Autodesk Fusion 360 part; units mm, degrees
sketch "Sketch1" plane through (0, 0, 0) normal (0, 0, 1) x (1, 0, 0)
  line L0 (0, 0) -> (49, 0)
  line L1 (49, 0) -> (49, 74)
  line L2 (49, 74) -> (0, 74)
  line L3 (0, 74) -> (0, 0)
extrude "Extrude1" add sketch "Sketch1" along normal blind 10
sketch "Sketch2" plane through (0, 0, 10) normal (0, 0, 1) x (-1, 0, 0)
  line L0 (0, -74) -> (0, 0)
  line L1 (0, 0) -> (-49, 0)
  line L2 (-49, 0) -> (-49, -74)
  line L3 (-49, -74) -> (0, -74)
  line L4 (-1.9, -72.1) -> (-47.1, -72.1)
  line L5 (-47.1, -72.1) -> (-47.1, -1.9)
  line L6 (-47.1, -1.9) -> (-1.9, -1.9)
  line L7 (-1.9, -1.9) -> (-1.9, -72.1)
extrude "Extrude2" cut sketch "Sketch2" against normal blind 9 contours L4 L5 L6 L7
sketch "Sketch3" plane through (0, 74, 0) normal (0, 1, 0) x (-1, 0, 0)
  line L0 (-49, 0) -> (0, 0)
  line L1 (0, 0) -> (0, 10)
  line L2 (0, 10) -> (-49, 10)
  line L3 (-49, 10) -> (-49, 0)
sketch "Sketch4" plane through (0, 74, 0) normal (0, 1, 0) x (-1, 0, 0)
  line L0 (-5, 5) -> (-19, 5)
  line L1 (-19, 5) -> (-19, 10)
  line L2 (-19, 10) -> (-5, 10)
  line L3 (-5, 10) -> (-5, 5)
extrude "Extrude3" cut sketch "Sketch4" against normal blind 6
sketch "Sketch5" plane through (0, 0, 0) normal (0, 1, 0) x (1, 0, 0)
sketch "Sketch6" plane through (0, 0, 0) normal (0, -1, 0) x (1, 0, 0)
  line L0 (0, 0) -> (49, 0)
  line L1 (49, 0) -> (49, 10)
  line L2 (49, 10) -> (0, 10)
  line L3 (0, 10) -> (0, 0)
  line L4 (6, 5) -> (19, 5)
  line L5 (19, 5) -> (19, 10)
  line L6 (19, 10) -> (6, 10)
  line L7 (6, 10) -> (6, 5)
extrude "Extrude4" cut sketch "Sketch6" against normal blind 6 contours L2 L4 L5 L6 L7
sketch "Sketch7" plane through (0, 0, 0) normal (-1, 0, 0) x (0, -1, 0)
  line L0 (-74, 0) -> (0, 0)
  line L1 (0, 0) -> (0, 10)
  line L2 (0, 10) -> (-74, 10)
  line L3 (-74, 10) -> (-74, 0)
  line L4 (-23, 11) -> (-47, 11)
  line L5 (-47, 11) -> (-47, 3)
  line L6 (-47, 3) -> (-23, 3)
  line L7 (-23, 3) -> (-23, 11)
extrude "Extrude5" cut sketch "Sketch7" against normal blind 3 contours L2 L5 L6 L7
sketch "Sketch8" plane through (0, 0, 1) normal (0, 0, 1) x (-1, 0, 0)
  line L0 (-1.9, -1.9) -> (-47.1, -1.9)
  line L1 (-47.1, -1.9) -> (-47.1, -72.1)
  line L2 (-47.1, -72.1) -> (-1.9, -72.1)
  line L3 (-1.9, -72.1) -> (-1.9, -1.9)
  line L4 (-4.05, -50) -> (-8, -50)
  line L5 (-8, -50) -> (-8, -49.05)
  line L6 (-8, -49.05) -> (-4.05, -49.05)
  line L7 (-4.05, -49.05) -> (-4.05, -50)
  line L8 (-7, -49.05) -> (-8, -49.05)
  line L9 (-8, -49.05) -> (-8, -45.05)
  line L10 (-8, -45.05) -> (-7, -45.05)
  line L11 (-7, -45.05) -> (-7, -49.05)
  line L12 (-7, -45.05) -> (-4.05, -45.05)
  line L13 (-4.05, -45.05) -> (-4.05, -45.95)
  line L14 (-4.05, -45.95) -> (-7, -45.95)
  line L15 (-7, -45.95) -> (-7, -45.05)
  line L16 (-7, -47.05) -> (-5.05, -47.05)
  line L17 (-5.05, -47.05) -> (-5.05, -47.95)
  line L18 (-5.05, -47.95) -> (-7, -47.95)
  line L19 (-7, -47.95) -> (-7, -47.05)
  line L20 (-44.95, -50) -> (-41, -50)
  line L21 (-41, -50) -> (-41, -49.05)
  line L22 (-41, -49.05) -> (-44.95, -49.05)
  line L23 (-44.95, -49.05) -> (-44.95, -50)
  line L24 (-41, -49.05) -> (-42, -49.05)
  line L25 (-42, -49.05) -> (-42, -45)
  line L26 (-42, -45) -> (-41, -45)
  line L27 (-41, -45) -> (-41, -49.05)
  line L28 (-42, -47.95) -> (-43.95, -47.95)
  line L29 (-43.95, -47.95) -> (-43.95, -47.05)
  line L30 (-43.95, -47.05) -> (-42, -47.05)
  line L31 (-42, -47.05) -> (-42, -47.95)
  line L32 (-42, -45) -> (-44.95, -45)
  line L33 (-44.95, -45) -> (-44.95, -45.95)
  line L34 (-44.95, -45.95) -> (-42, -45.95)
  line L35 (-42, -45.95) -> (-42, -45)
extrude "Extrude6" add sketch "Sketch8" along normal blind 35 contours L4 L5 L6 L7 L8 | L6 L8 L9 L10 L11 L15 L19 | L11 L16 L17 L18 L19 | L11 L12 L13 L14 L15 | L20 L21 L22 L23 L24 | L22 L24 L25 L26 L27 L31 L35 | L25 L28 L29 L30 L31 | L25 L32 L33 L34 L35
sketch "Sketch9" plane through (0, 0, 0) normal (-1, 0, 0) x (0, -1, 0)
sketch "Sketch10" plane through (0, 0, 1) normal (0, 0, 1) x (-1, 0, 0)
  line L0 (-5.05, -47.95) -> (-7, -47.95)
  line L1 (-7, -47.95) -> (-7, -49.05)
  line L2 (-7, -49.05) -> (-4.05, -49.05)
  line L3 (-4.05, -49.05) -> (-4.05, -50)
  line L4 (-4.05, -50) -> (-8, -50)
  line L5 (-8, -50) -> (-8, -45.05)
  line L6 (-8, -45.05) -> (-4.05, -45.05)
  line L7 (-4.05, -45.05) -> (-4.05, -45.95)
  line L8 (-4.05, -45.95) -> (-7, -45.95)
  line L9 (-7, -45.95) -> (-7, -47.05)
  line L10 (-7, -47.05) -> (-5.05, -47.05)
  line L11 (-5.05, -47.05) -> (-5.05, -47.95)
  line L12 (-41, -45) -> (-41, -50)
  line L13 (-41, -50) -> (-44.95, -50)
  line L14 (-44.95, -50) -> (-44.95, -49.05)
  line L15 (-44.95, -49.05) -> (-42, -49.05)
  line L16 (-42, -49.05) -> (-42, -47.95)
  line L17 (-42, -47.95) -> (-43.95, -47.95)
  line L18 (-43.95, -47.95) -> (-43.95, -47.05)
  line L19 (-43.95, -47.05) -> (-42, -47.05)
  line L20 (-42, -47.05) -> (-42, -45.95)
  line L21 (-42, -45.95) -> (-44.95, -45.95)
  line L22 (-44.95, -45.95) -> (-44.95, -45)
  line L23 (-44.95, -45) -> (-41, -45)
  line L24 (-1.9, -1.9) -> (-47.1, -1.9)
  line L25 (-47.1, -1.9) -> (-47.1, -72.1)
  line L26 (-47.1, -72.1) -> (-1.9, -72.1)
  line L27 (-1.9, -72.1) -> (-1.9, -1.9)
  line L28 (-27.95, -4.05) -> (-27.05, -4.05)
  line L29 (-27.05, -4.05) -> (-27.05, -8)
  line L30 (-27.05, -8) -> (-27.95, -8)
  line L31 (-27.95, -8) -> (-27.95, -4.05)
  line L32 (-27.0625, -8) -> (-23.0375, -8)
  line L33 (-23.0375, -8) -> (-23.0375, -7)
  line L34 (-23.0375, -7) -> (-27.0625, -7)
  line L35 (-27.0625, -7) -> (-27.0625, -8)
  line L36 (-23.0375, -7) -> (-23.95, -7)
  line L37 (-23.95, -7) -> (-23.95, -4.05)
  line L38 (-23.95, -4.05) -> (-23.0375, -4.05)
  line L39 (-23.0375, -4.05) -> (-23.0375, -7)
  line L40 (-25.05, -7) -> (-25.95, -7)
  line L41 (-25.95, -7) -> (-25.95, -5.05)
  line L42 (-25.95, -5.05) -> (-25.05, -5.05)
  line L43 (-25.05, -5.05) -> (-25.05, -7)
extrude "Extrude7" add sketch "Sketch10" along normal blind 35 contours L28 L29 L30 L31 L34 L35 | L29 L32 L33 L34 L36 L40 | L29 L30 L32 L34 L35 | L34 L40 L41 L42 L43 | L34 L36 L37 L38 L39
Geometry check sheet. Reference: the model listing, model coordinates, mm. A direction names the side the tool comes from. Round coordinates to 2 decimals unless told otherwise and drop trailing zeros. Loops run counter-clockwise (first coordinate to the right, second up) from the corner with the lowest first, then second, coordinate; pieces in that order, holes last. Notation, with made-up numbers: M -32.5,66.5 L -28.5,66.5 A32 cw -28.5,105.5 Z; hole C 72,13.5 d1. An arc over 180 degrees is marked long. Return JSON: item names as keys, results as strings. Group by question number.
(1) Scan lines: line 1 along Y through (x, z) = (6, 2.5); line 2 along Y through (x, z) = (35, 7.5); line 3 along X through (y, z) = (43.5, 6.5). Record each from-to range of solid material in increasing order. Write a range as [from, to].
(2) Mould release check, pull along Y, two halves, no side actions. Record for faces 4 (the face through (25.5, 6.4, 36)), 5 (the face through (43, 45, 18)): pulls with the +Y half, pulls with the -Y half, needs draft (parallel to the pull), parting line crosses it, or undercut.
(3) Section check A-A, the plane x = 22. Enter the section's corners in (y, z), and give its area (3 significant figures).
(4) Go/stop test with flat-tipped pins: pin 1 (8 mm diameter, centred on x = 21.5, y = 44.5, fed in from +Z); pin 2 (1 mm diameter, centred on x = 10, y = 73, fed in from +Z); pin 3 (1.2 mm diameter, centred on y = 46.5, z = 23, fed in from -X). Record where each tip stops, or that it passes through.
(5) Set-up check for faces 1 (the face through (1.9, 36.5, 2.6)), 2 (the face through (1, 23, 6)), 3 (the face through (6, 1, 8)): record each of +Z, -Z, +X, -X, +Y, -Y from which the full face is reachable in a straight line by a thin tool's end or side.
(6) Section check B-B, the plane y = 40.5. Enter the section's corners in (x, z), and give its area (3 significant figures).
(7) Section check C-C, the plane z = 11.5. Give the number of separate pieces and of enclosed holes in the cut face, and give its area (3 significant figures).
Data:
{
 "1": {"line 1": "[0, 1.9], [45.05, 45.95], [47.05, 47.95], [49.05, 50], [72.1, 74]", "line 2": "[0, 1.9], [72.1, 74]", "line 3": "[47.1, 49]"},
 "2": {"face 4": "needs draft", "face 5": "undercut"},
 "3": {"outline": "M 0,0 L 74,0 L 74,10 L 72.1,10 L 72.1,1 L 1.9,1 L 1.9,10 L 0,10 Z", "area": "108 mm²"},
 "4": {"pin 1": "z = 1", "pin 2": "z = 5", "pin 3": "x = 4.05"},
 "5": {"face 1": "+Z", "face 2": "+Z, -X", "face 3": "+Z, -Y"},
 "6": {"outline": "M 0,0 L 49,0 L 49,10 L 47.1,10 L 47.1,1 L 1.9,1 L 1.9,3 L 0,3 Z", "area": "69.9 mm²"},
 "7": {"separate pieces": "3", "enclosed holes": "0", "area": "36.5 mm²"}
}
